Design review of the part built by this model. Coordinates are the model's own, in mm. A direction names the side the tool comes from. Coordinates: 2 decimals unless noted, no trailing zeros. Use a Markdown table: item, result.
Autodesk Inventor part; units mm, degrees
ref_plane "YZ Plane" through (0, 0, 0) normal (1, 0, 0) x (0, 1, 0)
ref_plane "XZ Plane" through (0, 0, 0) normal (0, 1, 0) x (-1, 0, 0)
ref_plane "XY Plane" through (0, 0, 0) normal (0, 0, 1) x (1, 0, 0)
sketch "Sketch1" plane through (0, 0, 0) normal (0, 0, 1) x (1, 0, 0)
  line L0 (-178.7298, 623.3432) -> (284.8202, 623.3432)
  line L1 (284.8202, 623.3432) -> (284.8202, -278.3568)
  line L2 (284.8202, -278.3568) -> (-178.7298, -278.3568)
  line L3 (-178.7298, -278.3568) -> (-178.7298, 623.3432)
  point P0 (0, 0)
  dimension "d0" = 901.7
  dimension "d1" = 463.55
extrude "Board" add sketch "Sketch1" along normal blind 19.05
sketch "Sketch6" plane through (0, 0, 0) normal (0, 0, -1) x (-1, 0, 0)
  line L0 (-284.8202, 483.6432) -> (178.7298, 483.6432)
  line L1 (178.7298, 483.6432) -> (178.7298, 464.5932)
  line L2 (178.7298, 464.5932) -> (-284.8202, 464.5932)
  line L3 (-284.8202, 464.5932) -> (-284.8202, 483.6432)
  line L4 (178.7298, 623.3432) -> (-284.8202, 623.3432)
  line L5 (178.7298, -278.3568) -> (178.7298, 623.3432)
  line L6 (-284.8202, 623.3432) -> (-284.8202, -278.3568)
  line L7 (-284.8202, 29.6182) -> (178.7298, 29.6182)
  line L8 (178.7298, 29.6182) -> (178.7298, 10.5682)
  line L9 (178.7298, 10.5682) -> (-284.8202, 10.5682)
  line L10 (-284.8202, 10.5682) -> (-284.8202, 29.6182)
  point P0 (0, 0)
  dimension "d30" = 19.05
  dimension "d37" = 434.975
  dimension "d119" = 139.7
extrude "Right Shelf Dados" cut sketch "Sketch6" against normal blind 6.35 contours L0 L1 L2 L3 | L7 L5 L9 L6
sketch "Sketch32" plane through (0, 0, 0) normal (0, 0, -1) x (-1, 0, 0)
  line L0 (-157.8202, -78.3318) -> (178.7298, -78.3318)
  line L1 (178.7298, -78.3318) -> (178.7298, -84.6818)
  line L2 (178.7298, -84.6818) -> (-157.8202, -84.6818)
  line L3 (-157.8202, -84.6818) -> (-157.8202, -78.3318)
  line L4 (-157.8202, -173.5818) -> (178.7298, -173.5818)
  line L5 (178.7298, -173.5818) -> (178.7298, -179.9318)
  line L6 (178.7298, -179.9318) -> (-157.8202, -179.9318)
  line L7 (-157.8202, -179.9318) -> (-157.8202, -173.5818)
  line L8 (-284.8202, 623.3432) -> (-284.8202, -278.3568)
  line L9 (178.7298, 623.3432) -> (178.7298, -278.3568)
  line L10 (-284.8202, -278.3568) -> (178.7298, -278.3568)
  point P0 (0, 0)
  point P1 (-284.8202, 10.5682)
  dimension "d142" = 88.9
  dimension "d143" = 6.35
  dimension "d146" = 336.55
  dimension "d167" = 127
  dimension "d170" = 98.425
extrude "Right Wine Rack Horizonal Dados" cut sketch "Sketch32" against normal blind 6.35
sketch "Sketch33" plane through (0, 0, 0) normal (0, 0, -1) x (-1, 0, 0)
  line L0 (178.7298, 10.5682) -> (-284.8202, 10.5682)
  line L1 (70.7798, 10.5682) -> (77.1298, 10.5682)
  line L2 (77.1298, 10.5682) -> (77.1298, -278.3568)
  line L3 (77.1298, -278.3568) -> (70.7798, -278.3568)
  line L4 (70.7798, -278.3568) -> (70.7798, 10.5682)
  line L5 (-157.8202, -84.6818) -> (-157.8202, -78.3318)
  line L6 (-284.8202, -278.3568) -> (178.7298, -278.3568)
  point P0 (0, 0)
  dimension "d149" = 6.35
  dimension "d168" = 228.6
extrude "Right Wine Rack Vertical Dado" cut sketch "Sketch33" against normal blind 6.35
sketch "Sketch7" plane through (0, 0, 19.05) normal (0, 0, 1) x (1, 0, 0)
  line L0 (-178.7298, 483.6432) -> (284.8202, 483.6432)
  line L1 (284.8202, 483.6432) -> (284.8202, 464.5932)
  line L2 (284.8202, 464.5932) -> (-178.7298, 464.5932)
  line L3 (-178.7298, 464.5932) -> (-178.7298, 483.6432)
  line L4 (284.8202, 483.6432) -> (-178.7298, 483.6432)
  line L5 (-178.7298, 464.5932) -> (284.8202, 464.5932)
  line L6 (284.8202, -278.3568) -> (284.8202, 623.3432)
  line L7 (-178.7298, 623.3432) -> (-178.7298, -278.3568)
  line L8 (-178.7298, 29.6182) -> (284.8202, 29.6182)
  line L9 (284.8202, 29.6182) -> (284.8202, 10.5682)
  line L10 (284.8202, 10.5682) -> (-178.7298, 10.5682)
  line L11 (-178.7298, 10.5682) -> (-178.7298, 29.6182)
  point P0 (0, 0)
  point P1 (284.8202, 20.0932)
  dimension "d36" = 434.975
extrude "Left Shelf Dados" cut sketch "Sketch7" against normal blind 6.35 contours L0 L1 L2 L3 | L8 L6 L10 L7
sketch "Sketch34" plane through (0, 0, 19.05) normal (0, 0, 1) x (1, 0, 0)
  line L0 (157.8202, -78.3318) -> (-178.7298, -78.3318)
  line L1 (-178.7298, -78.3318) -> (-178.7298, -84.6818)
  line L2 (-178.7298, -84.6818) -> (157.8202, -84.6818)
  line L3 (157.8202, -84.6818) -> (157.8202, -78.3318)
  line L4 (157.8202, -173.5818) -> (-178.7298, -173.5818)
  line L5 (-178.7298, -173.5818) -> (-178.7298, -179.9318)
  line L6 (-178.7298, -179.9318) -> (157.8202, -179.9318)
  line L7 (157.8202, -179.9318) -> (157.8202, -173.5818)
  line L8 (284.8202, -278.3568) -> (284.8202, 10.5682)
  line L9 (-178.7298, 10.5682) -> (-178.7298, 483.6432)
  line L10 (-178.7298, -278.3568) -> (284.8202, -278.3568)
  point P0 (0, 0)
  dimension "d153" = 6.35
  dimension "d155" = 88.9
  dimension "d164" = 127
  dimension "d171" = 98.425
extrude "Left Wine Rack Horizontal Dados" cut sketch "Sketch34" against normal blind 6.35
sketch "Sketch35" plane through (0, 0, 19.05) normal (0, 0, 1) x (1, 0, 0)
  line L0 (284.8202, 10.5682) -> (-178.7298, 10.5682)
  line L1 (-77.1298, 10.5682) -> (-70.7798, 10.5682)
  line L2 (-70.7798, 10.5682) -> (-70.7798, -278.3568)
  line L3 (-70.7798, -278.3568) -> (-77.1298, -278.3568)
  line L4 (-77.1298, -278.3568) -> (-77.1298, 10.5682)
  line L5 (157.8202, -78.3318) -> (157.8202, -84.6818)
  line L6 (-178.7298, -278.3568) -> (284.8202, -278.3568)
  point P0 (0, 0)
  dimension "d159" = 6.35
  dimension "d165" = 228.6
extrude "Left Wine Rack  Vertical Dado" cut sketch "Sketch35" against normal blind 6.35
sketch "Sketch10" plane through (0, 0, 19.05) normal (0, 0, 1) x (1, 0, 0)
  line L0 (284.8202, -278.3568) -> (-178.7298, -278.3568)
  line L1 (-172.3798, 623.3432) -> (-166.0298, 623.3432)
  line L2 (-166.0298, 623.3432) -> (-166.0298, -278.3568)
  line L3 (-166.0298, -278.3568) -> (-172.3798, -278.3568)
  line L4 (-172.3798, -278.3568) -> (-172.3798, 623.3432)
  line L5 (-178.7298, 464.5932) -> (-178.7298, 29.6182)
  line L6 (284.8202, 623.3432) -> (-178.7298, 623.3432)
  point P0 (0, 0)
  point P1 (-172.3798, -278.3568)
  dimension "d172" = 6.35
  dimension "d173" = 6.35
extrude "Vertical Wire Channel" cut sketch "Sketch10" against normal blind 6.35
sketch "Sketch12" plane through (-178.7298, -278.3568, 12.7) normal (-1, 0, 0) x (0, 0, 1)
  line L0 (-6.35, 742.95) -> (0, 742.95)
  line L1 (0, 742.95) -> (0, 749.3)
  line L2 (0, 749.3) -> (-6.35, 749.3)
  line L3 (-6.35, 749.3) -> (-6.35, 742.95)
  line L4 (0, 288.925) -> (0, 307.975)
  line L5 (-6.35, 742.95) -> (-12.7, 742.95)
  point P0 (0, 0)
  point P1 (0, 901.7)
  dimension "d51" = 6.35
extrude "Top Horizontal Wire Channel" cut sketch "Sketch12" against normal blind 12.7
sketch "Sketch36" plane through (0, 0, 0) normal (0, 0, -1) x (-1, 0, 0)
  line L0 (77.1298, -278.3568) -> (178.7298, -278.3568)
  line L1 (178.7298, -278.3568) -> (159.6798, -278.3568)
  line L2 (159.6798, -278.3568) -> (159.6798, -268.8318)
  line L3 (159.6798, -268.8318) -> (178.7298, -268.8318)
  line L4 (178.7298, -268.8318) -> (178.7298, -278.3568)
  point P0 (0, 0)
  dimension "d174" = 19.05
  dimension "d175" = 9.525
extrude "Extrusion33" cut sketch "Sketch36" against normal blind 19.05
properties part number "Vertical Shelf"
(1) Machinability: for faces 1 (the flat face through (56, 474, 6.35)), 2 (the flat face through (-129, -33, 0)), which of the approach directions +Z, -Z, +X, -X, +Y, -Y give a long, thin tool a straight path to every point of the face, cutting with its end or side? Answer none if there is none.
Determined:
| item | result |
|---|---|
| face 1 | -Z, +X, -X |
| face 2 | -Z, +X, -X, +Y, -Y |
(2) Take a section at A-A on z = 16. State how many separate pieces and enclosed holes the cut face has, and give its area (3 significant figures).
Determined:
| item | result |
|---|---|
| separate pieces | 11 |
| enclosed holes | 0 |
| area | 389,000 mm2 |
(3) For pin 1 (1.9 mm diameter, centred on y = -176.5, z = 17, fed in from -X); pin 2 (6 mm diameter, centred on x = -83.5, y = 180.5, fed in from -Z), all flat-tipped, find the tip position at first contact; note any pin that passes through.
Determined:
| item | result |
|---|---|
| pin 1 | x = 157.82 |
| pin 2 | z = 0 |
(4) Draft analysis for pull direction Y (two halves, no side actions). For faces 3 (the flat face through (-51, 12, 12.7)), 4 (the flat face through (-178.73, 93, 9)), 5 (the flat face through (66, -278.357, 9)), state which applies: +Y half, -Y half, draft (parallel to the pull), parting line (faces both ways), or undercut.
Determined:
| item | result |
|---|---|
| face 3 | undercut |
| face 4 | draft |
| face 5 | -Y half |
(5) For L1, parallel to Y at x = 232, z = 1.75; L2, parallel to Y at x = -9.5, z = 1.5; L3, parallel to X at y = 388, z = 13, list the stretches that pass through material, from the lowest coordinate up. Write a range as from..to.
Determined:
| item | result |
|---|---|
| L1 | -278.36..10.57, 29.62..464.59, 483.64..623.34 |
| L2 | -278.36..-179.93, -173.58..-84.68, -78.33..10.57, 29.62..464.59, 483.64..623.34 |
| L3 | -178.73..-172.38, -166.03..284.82 |
